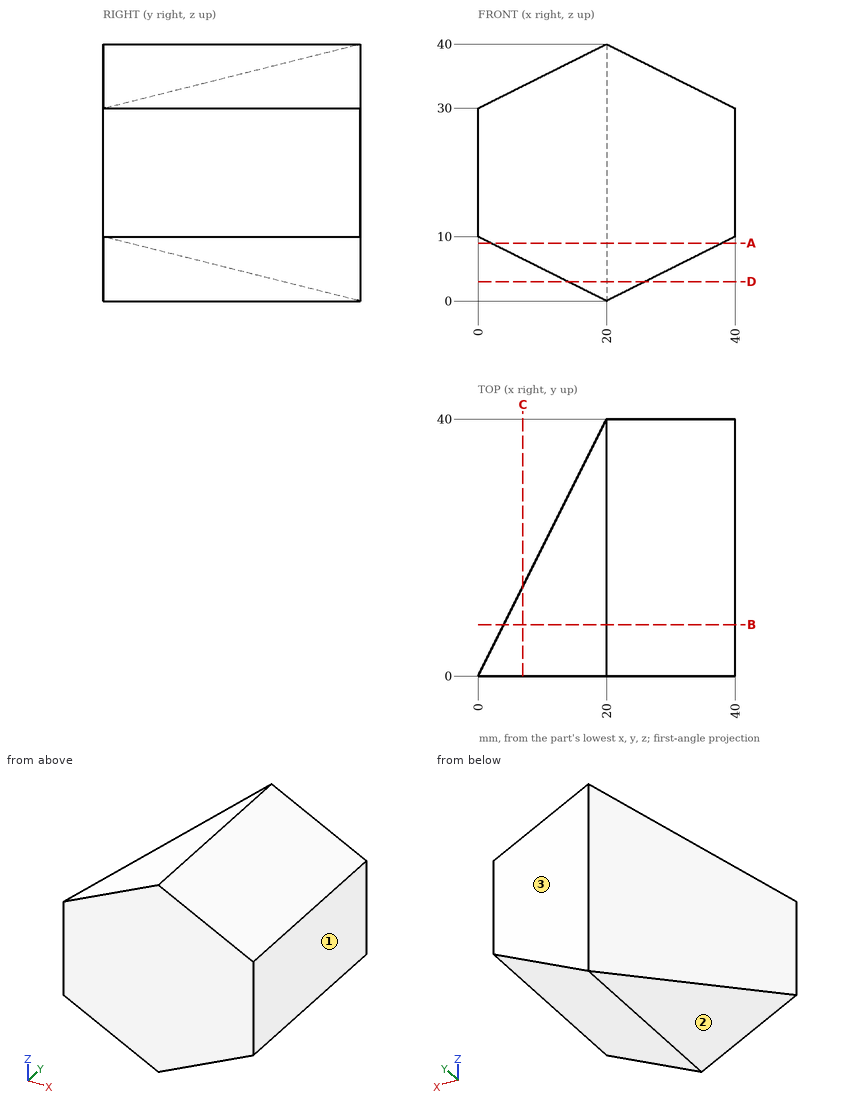
Study the drawing (mm; zero at the part's minimum x, y, z) and answer. Give positions to 0.01 mm unless a question says otherwise; leave off trailing zeros. Write each loop counter-clockwise with the first axis right and the second up, starting at its lowest first coordinate (ties: lowest second). Pieces come first, ordered by that corner, then holes. Notation, with made-up numbers: (18, -27.75) - (52, -27.75) arc R26 cw to (52, 4.25) - close; hole circle Ø7 at (-20.5, -38.75). An arc over 180 degrees is marked (long way). One line per question, with ' | ' between items. Start each with the question number.
1. Straight lines are drawn through the part: line 1 (X direction, y = 10.5, z = 37); line 2 (X direction, y = 8, z = 25); line 3 (Y direction, x = 13.5, z = 22.5). For each, find the intervals that lie inside material, in ascending order.
2. Section C-C, the plane x = 7 is taken. Determine the outline of the cut face in (y, z), then the cut area to 3 significant figures.
3. Section B-B, the plane y = 8 is taken. Determine the outline of the cut face in (x, z), then the cut area to 3 significant figures.
4. Given P1, Ø6, axis at x = 16.5, y = 16, coming from the +Z side; P2, Ø1.5, axis at x = 22.5, y = 16.5, coming from the -Z side (3 decimals); P3, Ø1.5, axis at x = 34.5, z = 16, coming from the -Y side; P4, Ø4, axis at x = 13.5, z = 28.5, coming from the +Y side, each flat-ended and moving along its own axis, determine where each tip first touches the part or whether it passes through.
5. Section D-D, the plane z = 3 is taken. Determine the outline of the cut face in (x, y), then the cut area to 3 significant figures.
6. Section A-A, the plane z = 9 is taken. Determine the outline of the cut face in (x, y).
7. Determine the mould class of the marked faces 1, 2 and 3 for opening direction X: +X half, -X half, draft (parallel to the pull), parting line (faces both ways), or undercut.
Result:
1) line 1: x = 14 to 26 | line 2: x = 4 to 40 | line 3: y = 0 to 27
2) outline: (0, 6.5) - (14, 6.5) - (14, 33.5) - (0, 33.5) - close | area: 378 mm2
3) outline: (4, 8) - (20, 0) - (40, 10) - (40, 30) - (20, 40) - (4, 32) - close | area: 1,110 mm2
4) P1: stops at z = 39.75 | P2: stops at z = 0.875 | P3: stops at y = 0 | P4: stops at y = 31
5) outline: (14, 0) - (26, 0) - (26, 40) - (20, 40) - (14, 28) - close | area: 444 mm2
6) outline: (2, 0) - (38, 0) - (38, 40) - (20, 40) - (2, 4) - close
7) face 1: +X half | face 2: -X half | face 3: draft
